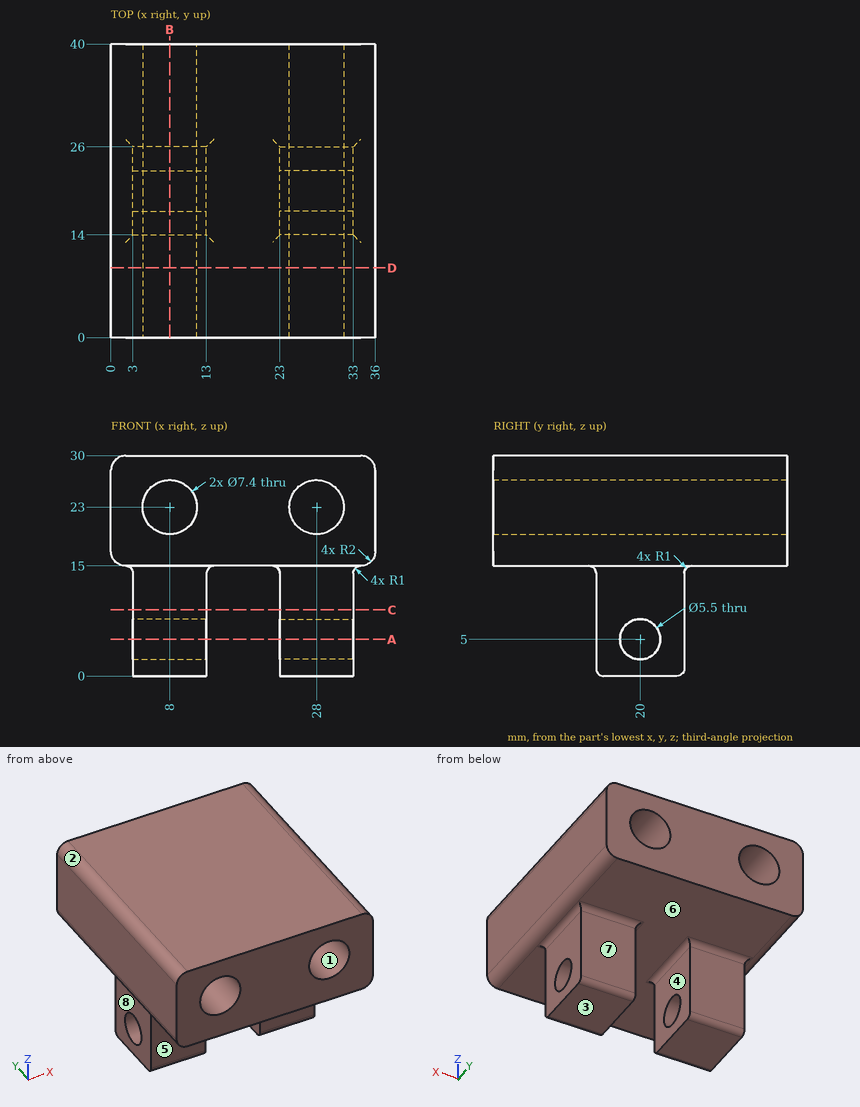
Geometry check sheet. Reference: drawing and pictorial views, mm from the part's lowest x, y, z. A direction names the side the tool comes from. Give positions to 0.01 mm unless a question says otherwise; leave off trailing zeros. Order: outer loops, then holes, each group sorted by start corner. A loop starts at its lowest first (then second) coordinate and runs counter-clockwise, first axis right, second up. Notation, with made-up numbers: M 40,-28.75 L 58,-28.75 A22 ccw 58,-5.75 Z; hole C 73.25,63 d10. An arc over 180 degrees is marked long. Use one line per item in the form item = value. Start each with the question number.
Q1. Section check D-D (y = 9.5). Enter the section's corners in (x, z).
Q2. Access from +Z, -Z, +X, -X, +Y, -Y to the whole of each face (thin tool, end or side, straight path). Record for the marked faces 5, 6, 7 and 8.
Q3. Section check A-A (z = 5). Enter the section's corners in (x, y).
Q4. Go/stop test with flat-tipped pins: pin 1 Ø11 at (x, z) = (28, 8.5) entering from -Y; pin 2 Ø9 at (y, z) = (20, 5) entering from -X; pin 3 Ø8 at (x, z) = (28, 7) entering from +Y. Record where each tip stops, or that it passes through.
Q5. Section check C-C (z = 9). Enter the section's corners in (x, y).
Q6. Mould release check, pull along X, two halves, no side actions. Record for the marked faces 1, 2, 3 and 4: +X half, -X half, draft (parallel to the pull), parting line (faces both ways), or undercut.
Q7. Section check B-B (x = 8). Enter the section's corners in (y, z).
Q8. Scan lines: line 1 along X through (y, z) = (17, 23); line 2 along Z through (x, y) = (28, 24.5); line 3 along X through (y, z) = (15, 7). Record each from-to range of solid material in increasing order. Write a range as [from, to].
Evaluation:
q1.outline = M 0,17 A2 ccw 2,15 L 34,15 A2 ccw 36,17 L 36,28 A2 ccw 34,30 L 2,30 A2 ccw 0,28 Z; hole C 8,23 d7.4; hole C 28,23 d7.4
q2.face_5 = -Z, +X, -X, -Y
q2.face_6 = -Z
q2.face_7 = -Z, +X, -X, +Y
q2.face_8 = -Z, -X, +Y, -Y
q3.outline = M 3,14 L 13,14 L 13,17.25 L 3,17.25 Z; M 3,22.75 L 13,22.75 L 13,26 L 3,26 Z; M 23,14 L 33,14 L 33,17.25 L 23,17.25 Z; M 23,22.75 L 33,22.75 L 33,26 L 23,26 Z
q4.pin_1 = 14
q4.pin_2 = 3
q4.pin_3 = 26
q5.outline = M 3,14 L 13,14 L 13,26 L 3,26 Z; M 23,14 L 33,14 L 33,26 L 23,26 Z
q6.face_1 = undercut
q6.face_2 = -X half
q6.face_3 = draft
q6.face_4 = undercut
q7.outline = M 0,15 L 13,15 A1 cw 14,14 L 14,1 A1 ccw 15,0 L 25,0 A1 ccw 26,1 L 26,14 A1 cw 27,15 L 40,15 L 40,19.3 L 0,19.3 Z; M 0,26.7 L 40,26.7 L 40,30 L 0,30 Z; hole C 20,5 d5.5
q8.line_1 = [0, 4.3], [11.7, 24.3], [31.7, 36]
q8.line_2 = [0, 19.3], [26.7, 30]
q8.line_3 = [3, 13], [23, 33]
